```python
from build123d import *
from OCP.BRepFilletAPI import BRepFilletAPI_MakeChamfer

# Parameters (mm, degrees)
BOSS_EXTRUDE1_DEPTH = 12.7
FILLET1_R           = 50
FILLET2_R           = 20
CUT_EXTRUDE1_DEPTH  = 261.135137957
CHAMFER1_SIZE       = 15
CHAMFER1_SIZE2      = 0.523811542
FILLET3_R           = 1
LPATTERN1_COUNT     = 3
LPATTERN1_PITCH     = 45.77
CUT_EXTRUDE2_DEPTH  = 261.135137957


with BuildPart() as part:
    # Sketch1 → Boss-Extrude1 (new body)
    with BuildSketch(Plane.XY):
        with BuildLine():
            Line((105, 153), (105, 103))
            ThreePointArc((105, 103), (124.067004371, 44.843678649), (180, 20))
            Line((180, 20), (210, 20))
            Line((210, 20), (210, 0))
            Line((210, 0), (171.4, 0))
            ThreePointArc((171.4, 0), (168.2, 3.2), (165, 0))
            Line((165, 0), (165, -16.05))
            Line((165, -16.05), (135, -16.05))
            Line((135, -16.05), (135, 0))
            ThreePointArc((135, 0), (131.8, 3.2), (128.6, 0))
            Line((128.6, 0), (116.4, 0))
            ThreePointArc((116.4, 0), (113.2, 3.2), (110, 0))
            Line((110, 0), (110, -16.05))
            Line((110, -16.05), (80, -16.05))
            Line((80, -16.05), (80, 0))
            Line((80, 0), (80, 153))
            Line((80, 153), (105, 153))
        make_face()
    extrude(amount=BOSS_EXTRUDE1_DEPTH)

    # Fillet1
    fillet1_edges = [part.edges().sort_by_distance(p)[0] for p in [
        (105, 103, 6.35),
    ]]
    fillet(fillet1_edges, radius=FILLET1_R)

    # Fillet2
    fillet2_edges = [part.edges().sort_by_distance(p)[0] for p in [
        (105, 153, 6.35),
    ]]
    fillet(fillet2_edges, radius=FILLET2_R)

    # Sketch2 → Cut-Extrude1 (cut, through all)
    with BuildSketch(Plane.XY.offset(12.7)):
        with BuildLine():
            Line((83.6, 15.7), (80, 15.7))
            Line((80, 15.7), (80, 3))
            Line((80, 3), (83.6, 3))
            ThreePointArc((83.6, 3), (86.8, -0.2), (90, 3))
            Line((90, 3), (90, 15.7))
            ThreePointArc((90, 15.7), (86.8, 18.9), (83.6, 15.7))
        make_face()
    cut_extrude1 = extrude(amount=-CUT_EXTRUDE1_DEPTH, mode=Mode.SUBTRACT)

    # Chamfer1: one chamfer whose edges measure the first distance from different faces: ONE call of the kernel's chamfer builder (chamfer() names one face for all edges)
    chamfer1_edges_1 = [part.edges().sort_by_distance(p)[0] for p in [
        (165, -16.05, 6.35),
    ]]
    chamfer1_side_1 = [part.faces().sort_by_distance(p)[0] for p in [
        (165, -8.025, 6.35),
    ]]
    chamfer1_edges_2 = [part.edges().sort_by_distance(p)[0] for p in [
        (135, -16.05, 6.35),
    ]]
    chamfer1_side_2 = [part.faces().sort_by_distance(p)[0] for p in [
        (135, -8.025, 6.35),
    ]]
    chamfer1_edges_3 = [part.edges().sort_by_distance(p)[0] for p in [
        (110, -16.05, 6.35),
    ]]
    chamfer1_side_3 = [part.faces().sort_by_distance(p)[0] for p in [
        (110, -8.025, 6.35),
    ]]
    chamfer1_edges_4 = [part.edges().sort_by_distance(p)[0] for p in [
        (80, -16.05, 6.35),
    ]]
    chamfer1_side_4 = [part.faces().sort_by_distance(p)[0] for p in [
        (80, -6.525, 6.35),
    ]]
    chamfer1 = BRepFilletAPI_MakeChamfer(part.part.solid().wrapped)
    for e in chamfer1_edges_1:
        chamfer1.Add(CHAMFER1_SIZE, CHAMFER1_SIZE2, e.wrapped, chamfer1_side_1[0].wrapped)  # the first distance lies on this face
    for e in chamfer1_edges_2:
        chamfer1.Add(CHAMFER1_SIZE, CHAMFER1_SIZE2, e.wrapped, chamfer1_side_2[0].wrapped)  # the first distance lies on this face
    for e in chamfer1_edges_3:
        chamfer1.Add(CHAMFER1_SIZE, CHAMFER1_SIZE2, e.wrapped, chamfer1_side_3[0].wrapped)  # the first distance lies on this face
    for e in chamfer1_edges_4:
        chamfer1.Add(CHAMFER1_SIZE, CHAMFER1_SIZE2, e.wrapped, chamfer1_side_4[0].wrapped)  # the first distance lies on this face
    add(Compound.cast(chamfer1.Shape()), mode=Mode.REPLACE)

    # Fillet3
    fillet3_edges = [part.edges().sort_by_distance(p)[0] for p in [
        (171.4, 0, 6.35),
        (128.6, 0, 6.35),
        (116.4, 0, 6.35),
        (83.6, 3, 6.35),
        (83.6, 15.7, 6.35),
        (109.476188458, -16.05, 6.35),
        (80.523811542, -16.05, 6.35),
        (135.523811542, -16.05, 6.35),
        (164.476188458, -16.05, 6.35),
    ]]
    fillet(fillet3_edges, radius=FILLET3_R)

    # LPattern1: Cut-Extrude1 ×3
    with Locations(*[(0, i * LPATTERN1_PITCH, 0) for i in range(1, LPATTERN1_COUNT)]):
        add(cut_extrude1, mode=Mode.SUBTRACT)

    # Sketch3 → Cut-Extrude2 (cut, through all)
    with BuildSketch(Plane.XY.offset(12.7)):
        with BuildLine():
            Line((80, 133.95), (90, 133.95))
            ThreePointArc((90, 133.95), (93.2, 137.15), (90, 140.35))
            Line((90, 140.35), (90, 153))
            Line((90, 153), (80, 153))
            Line((80, 153), (80, 133.95))
        make_face()
    extrude(amount=-CUT_EXTRUDE2_DEPTH, mode=Mode.SUBTRACT)


solid = part.part
```
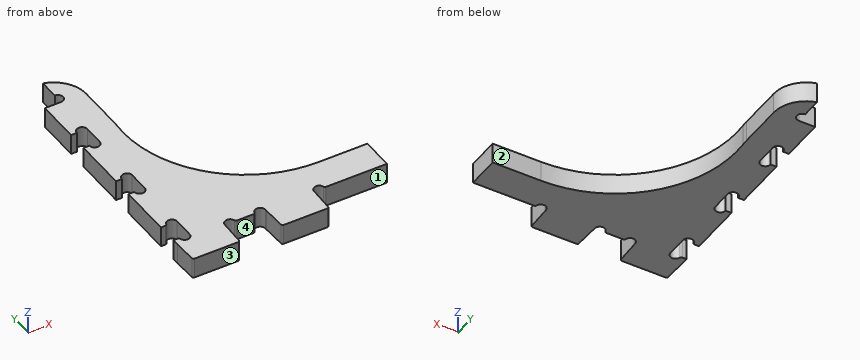
Model file for the job. Use its own axes, mm. Face numbers are marked on the shaded views. A direction names the side the tool comes from. Round coordinates to 2 decimals unless told otherwise and drop trailing zeros. Write each loop counter-clockwise with the first axis right and the second up, starting at its lowest first coordinate (ties: lowest second). Pieces come first, ordered by that corner, then holes. Notation, with made-up numbers: M 41,-20.5 L 60,-20.5 A21 cw 60,-10.5 Z; hole C -16.75,-21.75 d10. An arc over 180 degrees is marked long. Put each result on its own line as item: value.
Item 1: Probe L1, parallel to Y at x = 87.5, z = 10.5; L2, parallel to Y at x = 193, z = 1; L3, parallel to X at y = 107, z = 10.5. List the from-to ranges inside material, lowest first. Write a range as from..to.
Responses:
L1: -16.05..-0.12, 18.82..45.65, 64.59..91.42, 110.36..133.95
L2: 0..20
L3: 90..105
Item 2: Cut at B-B (y = 114). List the corners of the cut face in (x, z).
Responses:
outline: M 80,0 L 105,0 L 105,12.7 L 80,12.7 Z
Item 3: Cut at C-C (x = 142). List the corners of the cut face in (y, z).
Responses:
outline: M -16.05,0 L 30.28,0 L 30.28,12.7 L -16.05,12.7 Z
Item 4: Cut at A-A (x = 86.8). List the corners of the cut face in (y, z), and give its area (3 significant figures).
Responses:
outline: M -16.05,0 L -0.2,0 L -0.2,12.7 L -16.05,12.7 Z; M 18.9,0 L 45.57,0 L 45.57,12.7 L 18.9,12.7 Z; M 64.67,0 L 91.34,0 L 91.34,12.7 L 64.67,12.7 Z; M 110.44,0 L 133.95,0 L 133.95,12.7 L 110.44,12.7 Z
area: 1,180 mm²
Item 5: Tool access for the marked faces 1, 2, 3 and 4: list every direction of +Z, -Z, +X, -X, +Y, -Y with a clear straight run to the whole face (end or side of a thin tool).
Responses:
face 1: +Z, -Z, +X, -Y
face 2: +Z, -Z, +X, +Y
face 3: +Z, -Z, +X, -X, -Y
face 4: +Z, -Z, -Y
Item 6: Flat gauge pins, fed straight in: P1, Ø6.5, axis at y = 99, z = 7.5, coming from the -X side; P2, Ø1.5, axis at x = 109, y = 7.5, coming from the -Z side; P3, Ø0.5, axis at y = -0.5, z = 8, coming from the +X side; P4, Ø1, axis at x = 119, z = 5, coming from the +Y side. Where does each tip first touch, or does it go through?
Responses:
P1: x = 90
P2: z = 0
P3: x = 165
P4: y = 51.79
